Job drawing, mm, ordinate dimensions from the low corner. One solid piece. A direction names the side the tool comes from. Give positions to 0.01 mm unless a question says otherwise; leave off trailing zeros. Loops run counter-clockwise (first coordinate to the right, second up) from the corner with the lowest first, then second, coordinate; pieces in that order, holes last.
Item 1: Saw through at D-D on x = 7. Give the cut face in (y, z).
Item 2: Mould opens along Y. For the marked faces 4, 5 and 6 say: released by +Y, released by -Y, zero draft, split by the parting line, or undercut.
Item 3: Drop flat-ended pins along their axis: P1, Ø2, axis at x = 7, z = 5, coming from the -Y side; P2, Ø5, axis at x = 24, z = 3.5, coming from the +Y side. Give the stop position or say it passes through.
Item 4: Saw through at B-B on y = 42.5. Give the cut face in (x, z).
Item 5: Probe probe 1 along Y at (x, z) = (21.5, 7); probe 2 along X at (y, z) = (40.5, 9.25); probe 3 along Z at (x, y) = (37, 6.5). List the from-to ranges inside material, lowest first.
Item 6: Saw through at C-C on z = 2.25. Give the cut face in (x, y).
Item 7: Which spindle directions (+Z, -Z, +X, -X, +Y, -Y) get a long thin tool onto all of the face, cutting with end or side? Do the marked faces 1, 2 and 3. Say none if no direction does.
Item 8: Saw through at A-A on x = 17. Give the cut face in (y, z), plus the area to 3 significant figures.
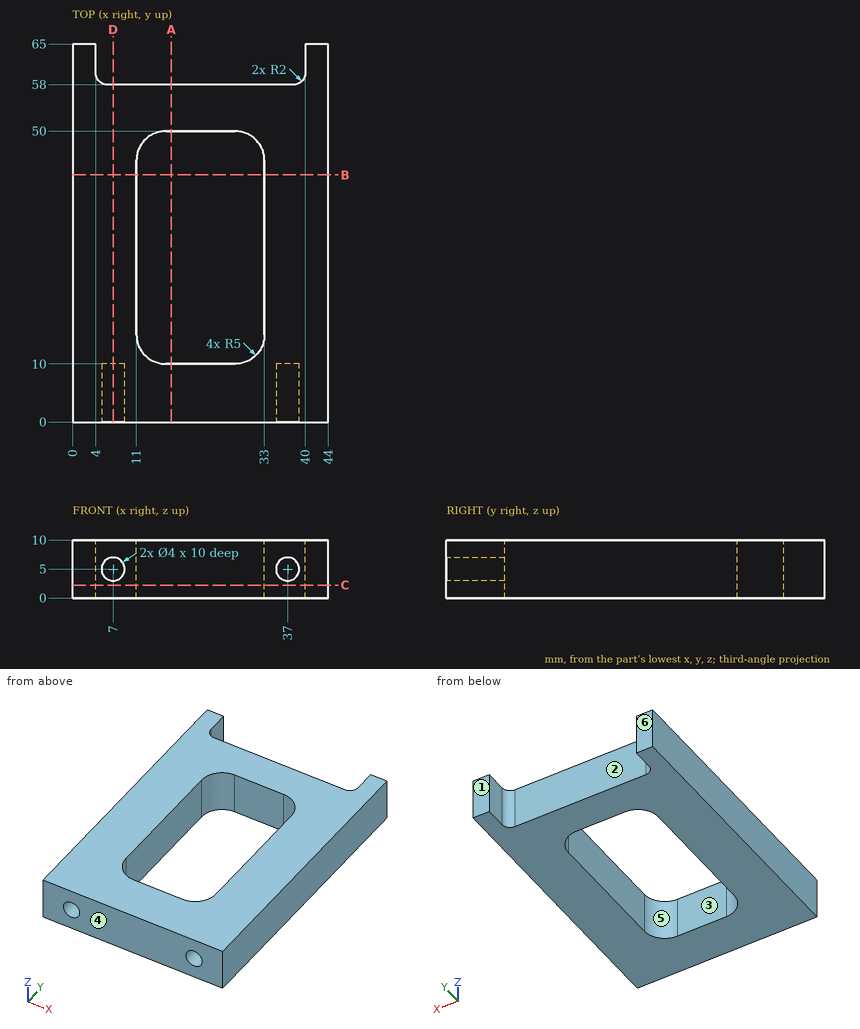
Results below:
1. outline: (0, 0) - (58, 0) - (58, 10) - (0, 10) - (0, 7) - (10, 7) - (10, 3) - (0, 3) - close
2. face 4: released by -Y
2. face 5: undercut
2. face 6: released by +Y
3. P1: stops at y = 10
3. P2: stops at y = 58
4. outline: (0, 0) - (11, 0) - (11, 10) - (0, 10) - close; (33, 0) - (44, 0) - (44, 10) - (33, 10) - close
5. probe 1: y = 0 to 10, 50 to 58
5. probe 2: x = 0 to 11, 33 to 44
5. probe 3: z = 0 to 3, 7 to 10
6. outline: (0, 0) - (44, 0) - (44, 65) - (40, 65) - (40, 60) arc R2 cw to (38, 58) - (6, 58) arc R2 cw to (4, 60) - (4, 65) - (0, 65) - close; hole (11, 15) arc R5 ccw to (16, 10) - (28, 10) arc R5 ccw to (33, 15) - (33, 45) arc R5 ccw to (28, 50) - (16, 50) arc R5 ccw to (11, 45) - close
7. face 1: +Z, -Z, +X, -X, +Y
7. face 2: +Z, -Z, +Y
7. face 3: +Z, -Z
8. outline: (0, 0) - (10, 0) - (10, 10) - (0, 10) - close; (50, 0) - (58, 0) - (58, 10) - (50, 10) - close
8. area: 180 mm2
